from build123d import *

# Parameters (mm, degrees)
F0_W     = 85
F0_H     = 80
F2_DEPTH = 25
F3_DEPTH = 5
F4_W     = 5
F4_H     = 61.4819614498
F5_DEPTH = 5


with BuildPart() as f2:
    # F0 (on Front) → F2 (new body)
    with BuildSketch(Plane.XZ):
        with Locations((1.5661627076, 1.7497490255)):
            Rectangle(F0_W, F0_H)
    extrude(amount=-F2_DEPTH)

    # F1 (on Front) → F3 (join)
    with BuildSketch(Plane.XZ):
        Polygon((-30.9338372924, -29.7322124243), (-30.9338372924, 31.7497490255), (-40.9338372924, 31.7497490255), (-40.9338372924, -38.2502509745), (44.0661627076, -38.2502509745), (44.0661627076, 31.7497490255), (34.0661627076, 31.7497490255), (34.0661627076, -29.7322124243), align=None)
    extrude(amount=F3_DEPTH)

    # F4 (on face) → F5 (join)
    with BuildSketch(Plane.XZ.offset(5)):
        with Locations((-28.4338372924, 1.0087683006)):
            Rectangle(F4_W, F4_H)
        Polygon((-30.9338372924, 31.7497490255), (-40.9338372924, 31.7497490255), (-40.9338372924, -38.2502509745), (44.0661627076, -38.2502509745), (44.0661627076, 31.7497490255), (34.0661627076, 31.7497490255), (34.0661627076, -29.7322124243), (29.0661627076, -29.7322124243), (-25.9338372924, -29.7322124243), (-30.9338372924, -29.7322124243), align=None)
        with Locations((31.5661627076, 1.0087683006)):
            Rectangle(F4_W, F4_H)
    extrude(amount=F5_DEPTH)


solid = f2.part
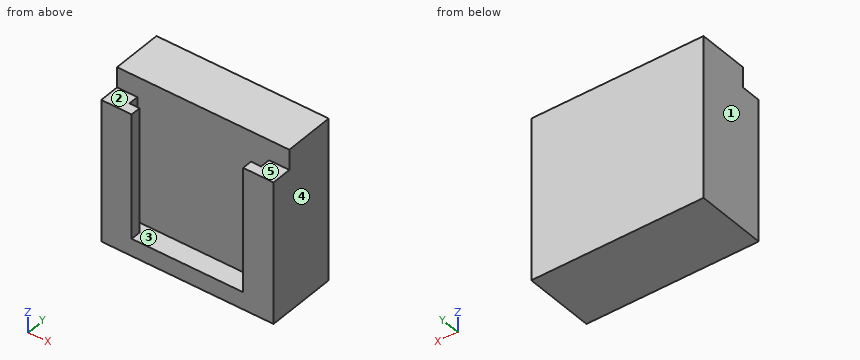
The model under review builds one solid part; all positions refer to its coordinate system, in mm. Face numbers are marked on the shaded views. A direction names the side the tool comes from. Give positions to 0.01 mm unless a question says otherwise; leave off trailing zeros. Write each loop counter-clockwise with the first axis right and the second up, starting at its lowest first coordinate (ties: lowest second). Pieces come first, ordered by that corner, then holes.
1. Draft analysis for pull direction X (two halves, no side actions). For the marked faces 1, 2 and 3, state which applies: +X half, -X half, draft (parallel to the pull), parting line (faces both ways), or undercut.
2. Tool access review of the marked faces 4 and 5: name each direction out of +Z, -Z, +X, -X, +Y, -Y from which nothing blocks a thin tool from reaching the whole face with its end or side.
3. For P1, Ø8, axis at x = 6, y = -5, coming from the +Z side; P2, Ø3, axis at x = 35.5, y = -4, coming from the +Z side; P3, Ø3, axis at x = -11.5, z = 11.5, coming from the -Y side, all flat-tipped, find the tip position at first contact; note any pin that passes through.
4. Add section B-B, the plane y = -4. Write out the cut boundary in (x, z).
5. Add section C-C, the plane x = 32.5. Write out the cut boundary in (y, z).
6. Add section D-D, the plane x = -21. Write out the cut boundary in (y, z), plus the area to 3 significant figures.
7. Add section A-A, the plane z = -8. Write out the cut boundary in (x, y), plus the area to 4 significant figures.
8. Wall thickness on L1, parallel to X at y = -4, z = 11; L2, parallel to X at y = -8, z = -24.5; L3, parallel to Y at x = -6, z = -12.5: over which ranges is each line inside the solid? List them lowest first.
Worked answers:
1. face 1: -X half
1. face 2: draft
1. face 3: undercut
2. face 4: +Z, -Z, +X, +Y, -Y
2. face 5: +Z, +X, -X, -Y
3. P1: stops at z = -29.73
3. P2: stops at z = 31.75
3. P3: stops at y = 0
4. outline: (-40.93, -38.25) - (44.07, -38.25) - (44.07, 31.75) - (34.07, 31.75) - (34.07, -29.73) - (-30.93, -29.73) - (-30.93, 31.75) - (-40.93, 31.75) - close
5. outline: (-10, -38.25) - (25, -38.25) - (25, 41.75) - (0, 41.75) - (0, -29.73) - (-5, -29.73) - (-5, 31.75) - (-10, 31.75) - close
6. outline: (-10, -38.25) - (25, -38.25) - (25, 41.75) - (0, 41.75) - (0, -29.73) - (-10, -29.73) - close
6. area: 2,090 mm2
7. outline: (-40.93, -10) - (-25.93, -10) - (-25.93, -5) - (-30.93, -5) - (-30.93, 0) - (34.07, 0) - (34.07, -5) - (29.07, -5) - (29.07, -10) - (44.07, -10) - (44.07, 25) - (-40.93, 25) - close
7. area: 2,375 mm2
8. L1: x = -40.93 to -30.93, 34.07 to 44.07
8. L2: x = -40.93 to -25.93, 29.07 to 44.07
8. L3: y = 0 to 25
